Model file for the job. Use its own axes, mm. A direction names the side the tool comes from. Coordinates: 2 decimals unless noted, no trailing zeros. Order: outer loops, then holes, each group sorted by start corner. A loop starts at its lowest first (then second) coordinate and runs counter-clockwise, first axis right, second up. Notation, with made-up numbers: M 51.5,-2.75 L 58.5,-2.75 A30 cw 58.5,21.25 Z; hole C -18,56.25 d10. An arc over 180 degrees is marked long. Return JSON: item names as keys, results as strings.
```python
from build123d import *

# Parameters (mm, degrees)
BOSS_EXTRUDE1_DEPTH      = 17
BOSS_EXTRUDE1_DEPTH_BACK = 17
SKETCH2_R                = 2.75
CUT_EXTRUDE1_DEPTH       = 9
SKETCH3_R                = 2.75
CUT_EXTRUDE2_DEPTH       = 9
SKETCH4_R                = 2.75
CUT_EXTRUDE3_DEPTH       = 9
SKETCH5_R                = 2.75
CUT_EXTRUDE4_DEPTH       = 9


with BuildPart() as part:
    # Sketch1 → Boss-Extrude1 (new body, two sides)
    with BuildSketch(Plane(origin=(0, 0, 0), x_dir=(0, 0, -1), z_dir=(1, 0, 0))) as boss_extrude1_sk:
        with BuildLine():
            Line((-50, 0), (-1, 0))
            ThreePointArc((-1, 0), (-0.292893219, 0.292893219), (0, 1))
            Line((0, 1), (0, 50))
            ThreePointArc((0, 50), (-0.292893219, 50.707106781), (-1, 51))
            Line((-1, 51), (-8, 51))
            ThreePointArc((-8, 51), (-8.707106781, 50.707106781), (-9, 50))
            Line((-9, 50), (-9, 31))
            Line((-9, 31), (-31, 9))
            Line((-31, 9), (-50, 9))
            ThreePointArc((-50, 9), (-50.707106781, 8.707106781), (-51, 8))
            Line((-51, 8), (-51, 1))
            ThreePointArc((-51, 1), (-50.707106781, 0.292893219), (-50, 0))
        make_face()
        with BuildLine():
            Line((-25.721825407, 5), (-20.999285733, 5))
            Line((-20.999285733, 5), (-16.494036438, 9.505249294))
            ThreePointArc((-16.494036438, 9.505249294), (-16.226979866, 9.987090789), (-16.255625497, 10.537245192))
            ThreePointArc((-16.255625497, 10.537245192), (-16.488859314, 11.683547702), (-16.418755424, 12.851234691))
            ThreePointArc((-16.418755424, 12.851234691), (-16.283360667, 13.048766752), (-16.046526031, 13.084263382))
            Line((-16.046526031, 13.084263382), (-14.300039569, 12.616293745))
            ThreePointArc((-14.300039569, 12.616293745), (-14.127781033, 12.492491496), (-14.080474622, 12.285701498))
            ThreePointArc((-14.080474622, 12.285701498), (-10.515075745, 10.515075774), (-12.285701539, 14.080474617))
            ThreePointArc((-12.285701539, 14.080474617), (-12.492491514, 14.127781045), (-12.616293745, 14.300039569))
            Line((-12.616293745, 14.300039569), (-13.084263382, 16.046526031))
            ThreePointArc((-13.084263382, 16.046526031), (-13.048766728, 16.283360705), (-12.851234602, 16.418755442))
            ThreePointArc((-12.851234602, 16.418755442), (-11.683774102, 16.488875269), (-10.537674556, 16.255773055))
            ThreePointArc((-10.537674556, 16.255773055), (-9.987311976, 16.226928716), (-9.505249294, 16.494036438))
            Line((-9.505249294, 16.494036438), (-5, 20.999285733))
            Line((-5, 20.999285733), (-5, 25.721825407))
            ThreePointArc((-5, 25.721825407), (-5.925974851, 27.107644706), (-7.560660172, 26.782485579))
            Line((-7.560660172, 26.782485579), (-26.782485579, 7.560660172))
            ThreePointArc((-26.782485579, 7.560660172), (-27.107644706, 5.925974851), (-25.721825407, 5))
        make_face(mode=Mode.SUBTRACT)
    extrude(amount=BOSS_EXTRUDE1_DEPTH)
    extrude(boss_extrude1_sk.sketch, amount=-BOSS_EXTRUDE1_DEPTH_BACK)

    # Sketch2 → Cut-Extrude1 (cut)
    with BuildSketch(Plane(origin=(0, 0, 0), x_dir=(-1, 0, 0), z_dir=(0, 1, 0))):
        with Locations((10, 41)):
            Circle(SKETCH2_R)
    extrude(amount=CUT_EXTRUDE1_DEPTH, mode=Mode.SUBTRACT)

    # Sketch3 → Cut-Extrude2 (cut)
    with BuildSketch(Plane(origin=(0, 0, 0), x_dir=(-1, 0, 0), z_dir=(0, 1, 0))):
        with Locations((-10, 41)):
            Circle(SKETCH3_R)
    extrude(amount=CUT_EXTRUDE2_DEPTH, mode=Mode.SUBTRACT)

    # Sketch4 → Cut-Extrude3 (cut)
    with BuildSketch(Plane.XY):
        with Locations((-10, 41)):
            Circle(SKETCH4_R)
    extrude(amount=CUT_EXTRUDE3_DEPTH, mode=Mode.SUBTRACT)

    # Sketch5 → Cut-Extrude4 (cut)
    with BuildSketch(Plane.XY):
        with Locations((10, 41)):
            Circle(SKETCH5_R)
    extrude(amount=CUT_EXTRUDE4_DEPTH, mode=Mode.SUBTRACT)


solid = part.part
```
Item 1: Wall check: line 1 (Z direction, x = -10, y = 3); line 2 (Y direction, x = 5, z = 12). Give the ranges that are in metal, low to high.
Check result:
{"line 1": "z = 0 to 38.25, 43.75 to 51", "line 2": "y = 0 to 9.9, 14.1 to 16.5, 22.34 to 28"}
Item 2: Drop flat-ended pins along their axis: pin 1 Ø3 at (x, z) = (10, 35) entering from +Y; pin 2 Ø4.5 at (x, y) = (-10, 41) entering from -Z; pin 3 Ø2.5 at (x, y) = (-5, 24) entering from +Z; pin 4 Ø9 at (x, y) = (10, 41) entering from +Z. Give the stop position or say it passes through.
Check result:
{"pin 1": "stops at y = 9", "pin 2": "passes through", "pin 3": "stops at z = 17.25", "pin 4": "stops at z = 9"}
Item 3: Pull direction Y, two halves, no side cores. Call faces 1 (the flat face through (0, 5, 51)), 2 (the flat face through (0, 20, 20)), 3 (the flat face through (0.238, 17.306, 17.037)): +Y half, -Y half, draft (parallel to the pull), parting line (faces both ways), or undercut.
Check result:
{"face 1": "draft", "face 2": "+Y half", "face 3": "undercut"}
Item 4: 3-axis set-ups, long thin cutter, end or side, ignore diameter. For faces 4 (the flat face through (0, 23, 5)), 5 (the flat face through (0, 41, 9)), 6 (the flat face through (0, 51, 4)): which of +Z, -Z, +X, -X, +Y, -Y reach the whole face in a straight line?
Check result:
{"face 4": "+X, -X", "face 5": "+Z, +X, -X, +Y", "face 6": "+Z, -Z, +X, -X, +Y"}
Item 5: Saw through at A-A (y = 41). Write the cut outline in (x, z), and give its area (3 significant figures).
Check result:
{"outline": "M -17,0 L -12.75,0 L -12.75,9 L -17,9 Z; M -7.25,0 L 7.25,0 L 7.25,9 L -7.25,9 Z; M 12.75,0 L 17,0 L 17,9 L 12.75,9 Z", "area": "207 mm2"}
Item 6: Saw through at D-D (x = 10). Count the separate pieces of the cut face and the enclosed holes in it, and give its area (3 significant figures).
Check result:
{"separate pieces": "3", "enclosed holes": "1", "area": "813 mm2"}
Item 7: Saw through at C-C (y = 6.5). Write the cut outline in (x, z), and give its area (3 significant figures).
Check result:
{"outline": "M -17,0 L 17,0 L 17,19.5 L -17,19.5 Z; M -17,27.22 L 17,27.22 L 17,51 L -17,51 Z; hole C -10,41 d5.5; hole C 10,41 d5.5", "area": "1,420 mm2"}
